```python
from build123d import *

# Parameters (mm, degrees)
IZIM1_W                       = 98.8
IZIM1_H                       = 74.5
TABAN_FLAN_1_DEPTH            = 3
KENAR_FLAN_1_STRIP_W          = 13.4732
KENAR_FLAN_1_STRIP_H          = 3
KENAR_FLAN_1_STRIP_CUT_DEPTH  = 65
KENAR_FLAN_1_RELIEF_W         = 14.9732
KENAR_FLAN_1_RELIEF_H         = 1.5
KENAR_FLAN_1_RELIEF_CUT_DEPTH = 3
KENAR_FLAN_1_DEPTH            = 65
IZIM9_R                       = 6.5
KES_EKSTR_ZYON1_DEPTH         = 10
IZIM11_R                      = 3.25
IZIM11_R_2                    = 3.166439954
KES_EKSTR_ZYON2_DEPTH         = 10


# Sheet-metal steps are written as plain solids
with BuildPart() as part:
    # Çizim1 → Taban-Flanş1 (new body)
    with BuildSketch(Plane.XY):
        Rectangle(IZIM1_W, IZIM1_H)
    extrude(amount=-TABAN_FLAN_1_DEPTH)

    # Kenar-Flanş1 strip (across the edge) → Kenar-Flanş1 strip cut (cut)
    with BuildSketch(Plane(origin=(-49.4, 32.5, 0), x_dir=(1, 0, 0), z_dir=(0, -1, 0))):
        with Locations((-6, -1.5)):
            Rectangle(KENAR_FLAN_1_STRIP_W, KENAR_FLAN_1_STRIP_H)
    extrude(amount=KENAR_FLAN_1_STRIP_CUT_DEPTH, mode=Mode.SUBTRACT)

    # Kenar-Flanş1 relief (on the sheet) → Kenar-Flanş1 relief cut (cut)
    with BuildSketch(Plane(origin=(-48.6634, 32.5, 0), x_dir=(1, 0, 0), z_dir=(0, 0, 1))):
        with Locations((-5.9866, 0.75)):
            Rectangle(KENAR_FLAN_1_RELIEF_W, KENAR_FLAN_1_RELIEF_H)
        with Locations((-5.9866, -65.75)):
            Rectangle(KENAR_FLAN_1_RELIEF_W, KENAR_FLAN_1_RELIEF_H)
    extrude(amount=-KENAR_FLAN_1_RELIEF_CUT_DEPTH, mode=Mode.SUBTRACT)

    # Kenar-Flanş1 section (across the edge) → Kenar-Flanş1 (add)
    with BuildSketch(Plane(origin=(-49.4, 32.5, 0), x_dir=(1, 0, 0), z_dir=(0, -1, 0))):
        with BuildLine():
            Line((-3, 0.7366), (-3, 55))
            Line((-3, 55), (0, 55))
            Line((0, 55), (0, 0.7366))
            ThreePointArc((0, 0.7366), (0.215745145, 0.215745145), (0.7366, 0))
            Line((0.7366, 0), (0.7366, -3))
            ThreePointArc((0.7366, -3), (-1.905575199, -1.905575199), (-3, 0.7366))
        make_face()
    extrude(amount=KENAR_FLAN_1_DEPTH)

    # Çizim9 → Kes-Ekstrüzyon1 (cut)
    with BuildSketch(Plane(origin=(-49.4, 0, 0), x_dir=(0, 0, -1), z_dir=(1, 0, 0))):
        with Locations((-26, 10.75)):
            Circle(IZIM9_R)
        with Locations((-26, -9.25)):
            Circle(IZIM9_R)
    extrude(amount=-KES_EKSTR_ZYON1_DEPTH, mode=Mode.SUBTRACT)

    # Çizim11 → Kes-Ekstrüzyon2 (cut)
    with BuildSketch(Plane.XY):
        with Locations((41.4, 28.25)):
            Circle(IZIM11_R)
        with Locations((-3.6, 28.25)):
            Circle(IZIM11_R)
        with Locations((-3.6, -26.75)):
            Circle(IZIM11_R)
        with Locations((41.4, -26.75)):
            Circle(IZIM11_R_2)
    extrude(amount=-KES_EKSTR_ZYON2_DEPTH, mode=Mode.SUBTRACT)


solid = part.part
```
Part model, mm, in its own coordinate system. A direction names the side the tool comes from. Give positions to 0.01 mm unless a question says otherwise; leave off trailing zeros. Write each loop counter-clockwise with the first axis right and the second up, starting at its lowest first coordinate (ties: lowest second). Pieces come first, ordered by that corner, then holes. Notation, with made-up numbers: M 87,-15.75 L 135,-15.75 A21 ccw 135,-7.75 Z; hole C -21.5,79 d5. An arc over 180 degrees is marked long. Use CSV: the item, a comma, the result in double quotes.
Item 1: Drill centre lines: probe 1 along Y at (x, z) = (-3.6, -0.65); probe 2 along Y at (x, z) = (41.4, -1.35); probe 3 along X at (y, z) = (-26, -1). Where is each one in solid material? Low to high.
Taken from the geometry:
probe 1,"y = -37.25 to -30, -23.5 to 25, 31.5 to 37.25"
probe 2,"y = -37.25 to -29.92, -23.58 to 25, 31.5 to 37.25"
probe 3,"x = -51.97 to -6.76, -0.44 to 38.32, 44.48 to 49.4"
Item 2: Slice it at A-A on y = -9.25. Write the cut outline in (x, z).
Taken from the geometry:
outline,"M -52.4,0.74 A3.74 ccw -48.66,-3 L 49.4,-3 L 49.4,0 L -48.66,0 A0.74 cw -49.4,0.74 L -49.4,19.5 L -52.4,19.5 Z; M -52.4,32.5 L -49.4,32.5 L -49.4,55 L -52.4,55 Z"
Item 3: Slice it at D-D on y = -26.75. Write the cut outline in (x, z), plus the area to 3 significant figures.
Taken from the geometry:
outline,"M -52.4,0.74 A3.74 ccw -48.66,-3 L -6.85,-3 L -6.85,0 L -48.66,0 A0.74 cw -49.4,0.74 L -49.4,55 L -52.4,55 Z; M -0.35,-3 L 38.23,-3 L 38.23,0 L -0.35,0 Z; M 44.57,-3 L 49.4,-3 L 49.4,0 L 44.57,0 Z"
area,"429 mm²"
Item 4: Which spindle directions (+Z, -Z, +X, -X, +Y, -Y) get a long thin tool onto all of the face, cutting with end or side? Do faces 4 (the face through (-49.4, 36, -1)), 5 (the face through (-1, 1, -3)), 6 (the face through (-49.4, 0, 28)), 7 (the face through (-48, 34, -1)), 8 (the face through (-49.4, -36, -1)). Say none if no direction does.
Taken from the geometry:
face 4,"+Z, -Z, -X, +Y"
face 5,"-Z, +X, -X, +Y, -Y"
face 6,"+Z, +X, +Y, -Y"
face 7,"+Z, -Z, -X"
face 8,"+Z, -Z, -X, -Y"
Item 5: Slice it at C-C on z = 26. Write the cut outline in (x, y), plus the area to 3 significant figures.
Taken from the geometry:
outline,"M -52.4,-32.5 L -49.4,-32.5 L -49.4,-15.75 L -52.4,-15.75 Z; M -52.4,-2.75 L -49.4,-2.75 L -49.4,4.25 L -52.4,4.25 Z; M -52.4,17.25 L -49.4,17.25 L -49.4,32.5 L -52.4,32.5 Z"
area,"117 mm²"
Item 6: Pull direction X, two halves, no side cores. Call faces 1 (the face through (-1, -37.25, -1)), 2 (the face through (43.1, -24.08, -1.48)), 3 (the face through (49.4, -1, -1)): +X half, -X half, draft (parallel to the pull), parting line (faces both ways), or undercut.
Taken from the geometry:
face 1,"draft"
face 2,"undercut"
face 3,"+X half"
Item 7: Pin check, flat tips, straight feed: P1, Ø6, axis at x = -49.5, z = 34, coming from the +Y side; P2, Ø1.5, axis at y = 35.5, z = -1, coming from the -X side; P3, Ø10.5, axis at y = 10.75, z = 26, coming from the -X side; P4, Ø1.2, axis at y = 33, z = -1, coming from the -X side. Stop position of each tip, or through.
Taken from the geometry:
P1,"stops at y = 32.5"
P2,"stops at x = -49.4"
P3,"passes through"
P4,"stops at x = -52.13"
Item 8: Slice it at B-B on x = -3.6. Write the cut outline in (y, z), plus the area to 4 significant figures.
Taken from the geometry:
outline,"M -37.25,-3 L -30,-3 L -30,0 L -37.25,0 Z; M -23.5,-3 L 25,-3 L 25,0 L -23.5,0 Z; M 31.5,-3 L 37.25,-3 L 37.25,0 L 31.5,0 Z"
area,"184.5 mm²"
